Work out the finished part from the listing and answer in its coordinate system (mm). A direction names the side the tool comes from. Round coordinates to 2 decimals unless told otherwise and drop trailing zeros. Order: outer loops, then holes, each group sorted by start corner. A loop starts at its lowest first (then second) coordinate and runs counter-clockwise, first axis right, second up. Notation, with made-up numbers: (45.5, 44) - (67.5, 44) arc R23 ccw to (67.5, 82) - close; hole circle Ø4 at (58.5, 22). An arc over 180 degrees is marked (long way). Put each result on its own line as item: value.
```python
from build123d import *

# Parameters (mm, degrees)
SKETCH1_W           = 63.5
SKETCH1_H           = 63.5
BOSS_EXTRUDE1_DEPTH = 5.334
SKETCH2_R           = 18.5
SKETCH2_W           = 12.7
SKETCH2_H           = 5.334
CUT_EXTRUDE1_DEPTH  = 5.334
SKETCH3_W           = 37
SKETCH3_H           = 32.300000043
CUT_EXTRUDE2_DEPTH  = 5.334


with BuildPart() as part:
    # Sketch1 → Boss-Extrude1 (new body)
    with BuildSketch(Plane.XY):
        with Locations((31.75, 31.75)):
            Rectangle(SKETCH1_W, SKETCH1_H)
    extrude(amount=BOSS_EXTRUDE1_DEPTH)

    # Sketch2 → Cut-Extrude1 (cut)
    with BuildSketch(Plane.XY.offset(5.334)):
        with Locations((31.75, 31.199999957)):
            Circle(SKETCH2_R)
        with Locations((19.05, 2.667)):
            Rectangle(SKETCH2_W, SKETCH2_H)
        with Locations((44.45, 2.667)):
            Rectangle(SKETCH2_W, SKETCH2_H)
    extrude(amount=-CUT_EXTRUDE1_DEPTH, mode=Mode.SUBTRACT)

    # Sketch3 → Cut-Extrude2 (cut)
    with BuildSketch(Plane.XY.offset(5.334)):
        with Locations((31.75, 47.349999979)):
            Rectangle(SKETCH3_W, SKETCH3_H)
    extrude(amount=-CUT_EXTRUDE2_DEPTH, mode=Mode.SUBTRACT)


solid = part.part
```
1) For faces 4 (the flat face through (7, 63.5, 3)), 5 (the flat face through (50.25, 47, 3)), 6 (the flat face through (50.8, 3, 3)), determine the directions among +Z, -Z, +X, -X, +Y, -Y from which every point of the face is accessible in a straight line to the end or side of a thin tool.
Findings below:
face 4: +Z, -Z, +X, -X, +Y
face 5: +Z, -Z, +Y
face 6: +Z, -Z, -Y
2) Given pin 1 Ø2.5 at (y, z) = (3, 3) entering from -X; pin 2 Ø2 at (x, z) = (27, 4) entering from +Y; pin 3 Ø2.5 at (x, z) = (17.5, 2.5) entering from -Y, each flat-ended and moving along its own axis, determine where each tip first touches the part or whether it passes through.
Findings below:
pin 1: stops at x = 0
pin 2: stops at y = 13.62
pin 3: stops at y = 5.33
3) A cutting plane is placed at D-D on y = 26. Write down the section's boundary in (x, z), then the cut area to 3 significant figures.
Findings below:
outline: (0, 0) - (14, 0) - (14, 5.33) - (0, 5.33) - close; (49.5, 0) - (63.5, 0) - (63.5, 5.33) - (49.5, 5.33) - close
area: 149 mm2
4) A cutting plane is placed at B-B on z = 3.05. Write down the section's boundary in (x, y), then the cut area to 3 significant figures.
Findings below:
outline: (0, 0) - (12.7, 0) - (12.7, 5.33) - (25.4, 5.33) - (25.4, 0) - (38.1, 0) - (38.1, 5.33) - (50.8, 5.33) - (50.8, 0) - (63.5, 0) - (63.5, 63.5) - (50.25, 63.5) - (50.25, 31.2) arc R18.5 cw to (13.25, 31.2) - (13.25, 63.5) - (0, 63.5) - close
area: 2,160 mm2
5) A cutting plane is placed at C-C on x = 31.75. Write down the section's boundary in (y, z).
Findings below:
outline: (0, 0) - (12.7, 0) - (12.7, 5.33) - (0, 5.33) - close
6) A cutting plane is placed at A-A on y = 39.5. Write down the section's boundary in (x, z), then the cut area to 3 significant figures.
Findings below:
outline: (0, 0) - (13.25, 0) - (13.25, 5.33) - (0, 5.33) - close; (50.25, 0) - (63.5, 0) - (63.5, 5.33) - (50.25, 5.33) - close
area: 141 mm2
7) Straight lines are drawn through the part: L1, parallel to X at y = 3.5, z = 4.2; L2, parallel to X at y = 36.5, z = 1.95; L3, parallel to Y at x = 25, z = 4.65. For each, find the intervals that lie inside material, in ascending order. Write a range as from..to.
Findings below:
L1: x = 0..12.7, 25.4..38.1, 50.8..63.5
L2: x = 0..13.25, 50.25..63.5
L3: y = 5.33..13.98
8) For a pull along X with two mould halves and no side action, classify faces 1 (the flat face through (31, 11, 0)), 2 (the flat face through (0, 31, 3)), 3 (the flat face through (19, 5.334, 3)) as pulls with the +X half, pulls with the -X half, needs draft (parallel to the pull), parting line crosses it, or undercut.
Findings below:
face 1: needs draft
face 2: pulls with the -X half
face 3: undercut
